Autodesk Inventor part; units mm, degrees
ref_plane "YZ Plane" through (0, 0, 0) normal (1, 0, 0) x (0, 1, 0)
ref_plane "XZ Plane" through (0, 0, 0) normal (0, 1, 0) x (-1, 0, 0)
ref_plane "XY Plane" through (0, 0, 0) normal (0, 0, 1) x (1, 0, 0)
sketch "Sketch1" plane through (0, 0, 0) normal (0, 0, 1) x (1, 0, 0)
  circle A0 centre (0, 0) radius 18.5
  line L0 (-15.5, 0) -> (15.5, 0)
  circle A1 centre (-15.5, 0) radius 1.7
  circle A2 centre (15.5, 0) radius 1.7
  dimension "d0" = 37
  dimension "d1" = 31
  dimension "d2" = 3.4
  dimension "d3" = 3.4
extrude "Extrusion1" add sketch "Sketch1" against normal blind 4.5
sketch "Sketch2" plane through (0, 0, 0) normal (0, 0, 1) x (1, 0, 0)
  arc A0 (8.4832, -8.4874) -> (-8.4832, -8.4874) centre (0, -9.9) ccw
  circle A1 centre (0, 0) radius 18.5
  circle A2 centre (0, -9.9) radius 6
  arc A3 (8.4832, -8.4874) -> (-8.4832, -8.4874) centre (0, 0) ccw
  arc A4 (-5.9787, -10.4045) -> (5.9787, -10.4045) centre (0, 0) ccw
  dimension "d10" = 17.2
  dimension "d11" = 12
extrude "Extrusion2" add sketch "Sketch2" along normal blind 6 contours A2 A4 | A4 A2
extrude "Extrusion3" cut sketch "Sketch2" against normal blind 1 contours A0 A3
sketch "Sketch3" plane through (0, -9.9, 6) normal (0, 0, 1) x (1, 0, 0)
  circle A0 centre (0, 0) radius 6
  circle A1 centre (0, 0) radius 3
  point P0 (0, 9.9)
  dimension "d16" = 6
extrude "Extrusion4" add sketch "Sketch3" along normal blind 15 contours A1
sketch "Sketch4" plane through (0, 0, -4.5) normal (0, 0, -1) x (-1, 0, 0)
  circle A0 centre (0, 0) radius 18.5
extrude "Extrusion5" add sketch "Sketch4" along normal blind 14.5
sketch "Sketch5" plane through (0, -9.9, 21) normal (0, 0, 1) x (1, 0, 0)
  circle A0 centre (0, 0) radius 3
  line L0 (1.2182, 2.7415) -> (1.2182, -2.7415)
  point P0 (0, 9.9)
extrude "Extrusion6" cut sketch "Sketch5" against normal blind 12 contours A0 L0 picked at (1.8121, 0)
sketch "Sketch6" plane through (0, 0, -19) normal (0, 0, -1) x (-1, 0, 0)
  circle A0 centre (0, 0) radius 16
  dimension "d23" = 32
extrude "Extrusion7" add sketch "Sketch6" along normal blind 22
sketch "Sketch7" plane through (0, 0, 0) normal (0, 0, 1) x (1, 0, 0)
  circle A0 centre (-15.5, 0) radius 1.7
  circle A1 centre (15.5, 0) radius 1.7
  circle A2 centre (0, 0) radius 18.5
properties part number "MOTOR DC"
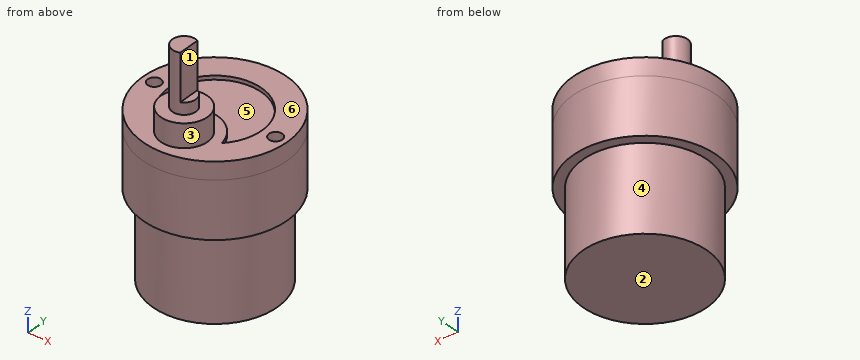
Source: CAD feature listing. Evaluate the final solid. Frame: model axes, mm. Face numbers are marked on the shaded views. A direction names the side the tool comes from. Coordinates: 2 decimals unless noted, no trailing zeros. Write each loop counter-clockwise with the first axis right and the second up, starting at its lowest first coordinate (ties: lowest second). Pieces come first, ordered by that corner, then holes. Notation, with made-up numbers: (35.25, 86.25) -> (52.25, 86.25) arc R21 cw to (52.25, 91.25) -> close; hole circle Ø3 at (86, 55). An arc over 180 degrees is marked (long way). Return JSON: item names as keys, results as strings. Group by question number.
1) Section query C-C, the plane z = -14. Return loops of the section in (x, y), plus the area to 3 significant figures.
2) Set-up query: the marked faces 1, 2 and 3. Return all of +Z, -Z, +X, -X, +Y, -Y with unobstructed straight access to the full face (end or side cutting, diameter ignored); none if empty.
3) Section query D-D, the plane x = 13. Return loops of the section in (y, z), plus the area to 3 significant figures.
4) Section query A-A, the plane x = 0. Return loops of the section in (y, z).
5) Ray query, line 1 along Z through (x, y) = (15, -0.5); line 2 along Z through (x, y) = (15.5, -9); line 3 along Y through (x, z) = (-15.5, -3.15). Return the intervals inside material, ascending.
6) Contact query for flat-ended pins moving along their axis: P1, Ø1, axis at y = -5.5, z = 4.5, coming from the +X side; P2, Ø2.5, axis at y = -10, z = 16, coming from the +X side; P3, Ø3, axis at x = -11, z = -25.5, coming from the +Y side. Output: stop coordinate, or through.
7) Section query B-B, the plane y = 0. Return loops of the section in (x, z), plus the area to 3 significant figures.
8) Mould query, pull axis X, two halves, no side actions, for the marked faces 4, 5 and 6. Classes: +X half, -X half, draft (parallel to the pull), parting line (faces both ways), or undercut.
From the geometry:
{
 "1": {"outline": "circle Ø37 at (0, 0)", "area": "1,080 mm²"},
 "2": {"face 1": "+Z, +X, +Y, -Y", "face 2": "-Z, +X, -X, +Y, -Y", "face 3": "+Z"},
 "3": {"outline": "(-13.16, -19) -> (-9.33, -19) -> (-9.33, -41) -> (9.33, -41) -> (9.33, -19) -> (13.16, -19) -> (13.16, 0) -> (-13.16, 0) -> close", "area": "911 mm²"},
 "4": {"outline": "(-18.5, -19) -> (-16, -19) -> (-16, -41) -> (16, -41) -> (16, -19) -> (18.5, -19) -> (18.5, 0) -> (12, 0) -> (12, -1) -> (-1.3, -1) -> (-1.3, 0) -> (-3.9, 0) -> (-3.9, 6) -> (-6.9, 6) -> (-6.9, 21) -> (-12.9, 21) -> (-12.9, 6) -> (-15.9, 6) -> (-15.9, 0) -> (-18.5, 0) -> close"},
 "5": {"line 1": "-41 to -4.5", "line 2": "-19 to 0", "line 3": "-10.1 to -1.7, 1.7 to 10.1"},
 "6": {"P1": "x = 4.56", "P2": "x = 1.22", "P3": "y = 12.87"},
 "7": {"outline": "(-18.5, -19) -> (-16, -19) -> (-16, -41) -> (16, -41) -> (16, -19) -> (18.5, -19) -> (18.5, 0) -> (17.2, 0) -> (17.2, -4.5) -> (13.8, -4.5) -> (13.8, 0) -> (12, 0) -> (12, -1) -> (-12, -1) -> (-12, 0) -> (-13.8, 0) -> (-13.8, -4.5) -> (-17.2, -4.5) -> (-17.2, 0) -> (-18.5, 0) -> close", "area": "1,350 mm²"},
 "8": {"face 4": "parting line", "face 5": "undercut", "face 6": "draft"}
}
